The model under review builds one solid part; all positions refer to its coordinate system, in mm. Round coordinates to 2 decimals unless told otherwise and drop trailing zeros. Order: outer loops, then holes, each group sorted by start corner. A loop starts at its lowest first (then second) coordinate and runs counter-clockwise, first axis right, second up. Notation, with made-up numbers: (39.5, -24.75) -> (88.5, -24.75) arc R19 cw to (88.5, -11.75) -> close; hole circle Ø4 at (56, 7.25). An arc over 180 degrees is marked (long way). Return JSON: item names as keys, results as strings. Group by question number.
Autodesk Inventor part; units mm, degrees
ref_plane "YZ Plane" through (0, 0, 0) normal (1, 0, 0) x (0, 1, 0)
ref_plane "XZ Plane" through (0, 0, 0) normal (0, 1, 0) x (-1, 0, 0)
ref_plane "XY Plane" through (0, 0, 0) normal (0, 0, 1) x (1, 0, 0)
sketch "Sketch1" plane through (0, 0, 0) normal (1, 0, 0) x (0, 1, 0)
  circle A0 centre (0, 0) radius 3
  dimension "d0" = 6
extrude "Extrusion1" add sketch "Sketch1" along normal blind 50.8
fillet "Fillet1" radius 1 1 edges at (50.8, -3, 0)
fillet "Fillet2" radius 1 1 edges at (0, -3, 0)
properties part number "axle small" material "Stainless Steel"
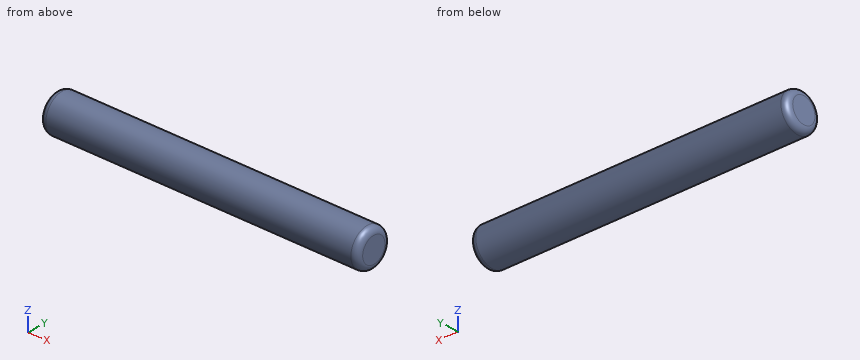
Item 1: Consider section A-A on x = 43.5. State the section outline as (y, z) points.
Item 2: Wall thickness on line 1 along X through (y, z) = (-0.2, 2.1); line 2 along Z through (x, y) = (32, -0.25); line 3 along Z through (x, y) = (45, 1): over which ranges is each line inside the solid? List them lowest first.
Item 3: Insertion check: pin 1 Ø1 at (x, z) = (37, -1.5) entering from -Y; pin 2 Ø2 at (x, z) = (40.5, -2.5) entering from -Y. Each pin has a flat end and moves straight along its axis. Give the tip position at first contact, or say it passes through.
Values:
{
 "1": {"outline": "circle Ø6 at (0, 0)"},
 "2": {"line 1": "0.01 to 50.79", "line 2": "-2.99 to 2.99", "line 3": "-2.83 to 2.83"},
 "3": {"pin 1": "y = -2.83", "pin 2": "y = -2.6"}
}
